Autodesk Inventor part; units mm, degrees
ref_plane "YZ Plane" through (0, 0, 0) normal (1, 0, 0) x (0, 1, 0)
ref_plane "XZ Plane" through (0, 0, 0) normal (0, 1, 0) x (-1, 0, 0)
ref_plane "XY Plane" through (0, 0, 0) normal (0, 0, 1) x (1, 0, 0)
sketch "Sketch1" plane through (0, 0, 0) normal (1, 0, 0) x (0, 1, 0)
  circle A0 centre (0, 0) radius 8.001
  dimension "d0" = 16.002
extrude "Extrusion1" add sketch "Sketch1" along normal blind 101.6254
sketch "Sketch2" plane through (101.6254, 0, 0) normal (1, 0, 0) x (0, 0, -1)
  line L0 (-6.2432, -5.0038) -> (6.2432, -5.0038)
  line L1 (-7.5991, -2.5038) -> (7.5991, -2.5038)
  arc A0 (6.2432, -5.0038) -> (7.5991, -2.5038) centre (0, 0) ccw
  arc A1 (-7.5991, -2.5038) -> (-6.2432, -5.0038) centre (0, 0) ccw
  circle A2 centre (0, 0) radius 8.001
  point P0 (7.0332, -3.8145)
  point P1 (-7.0332, -3.8145)
  dimension "d3" = 5.0038
  dimension "d4" = 2.5
extrude "Extrusion2" add sketch "Sketch2" along normal blind 22.86 contours A1 L1 A0 L0
sketch "Sketch3" plane through (101.6254, -2.5038, 7.5991) normal (0, 1, 0) x (1, 0, 0)
  circle A0 centre (15.2654, 7.5991) radius 4.1021
  line L0 (0, 15.1983) -> (22.86, 15.1983)
  line L1 (0, 0) -> (22.86, 0)
  line L2 (0, 0) -> (0, 15.1983)
  point P0 (-101.6254, 7.5991)
  dimension "d8" = 8.2042
  dimension "d9" = 7.5991
  dimension "d10" = 15.1983
  dimension "d13" = 15.2654
extrude "Extrusion3" cut sketch "Sketch3" against normal blind 15.0114
equation "\"d9\" = 0.5 * d10"
properties part number "Ring Connector model 5"
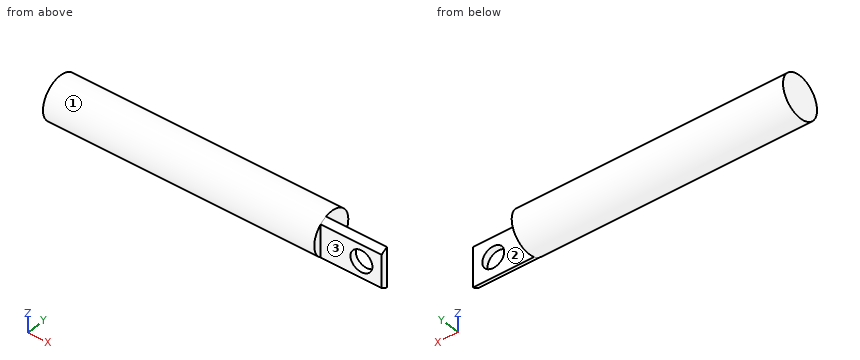
Geometry: final body of the model. Coordinates: model frame, mm. Face numbers are marked on the shaded views. A direction names the side the tool comes from. Give positions to 0.01 mm unless a question says otherwise; leave off trailing zeros. Write each loop counter-clockwise with the first axis right and the second up, starting at its lowest first coordinate (ties: lowest second). Pieces come first, ordered by that corner, then holes.
(1) First-contact query: P1, Ø7.5, axis at x = 117.5, z = 1.5, coming from the +Y side; P2, Ø1.5, axis at x = 65.5, z = 3.5, coming from the +Y side; P3, Ø2, axis at x = 12.5, y = -4, coming from the +Z side. Flat tips, straight axial feed; report the tip coordinate or a pass-through.
(2) Cut plane B-B, the plane x = 108. Return loops of the section in (y, z), then the cut area to 3 significant figures.
(3) Ray query, line 1 (X direction, y = -3.45, z = 0); line 2 (Z direction, x = 73, y = 5); line 3 (Z direction, x = 24.5, y = 0.5). Return the intervals inside material, ascending.
(4) Access query for the marked faces 1, 2 and 3. Directions: +Z, -Z, +X, -X, +Y, -Y. A direction counts if a zero-diameter tool reaches every point of the face in a straight line with its end or side. Return the directions, or none.
(5) Cut plane A-A, the plane z = 0. Return loops of the section in (x, y).
(6) Cut plane D-D, the plane x = 39. Return loops of the section in (y, z), then the cut area to 3 significant figures.
(7) Cut plane C-C, the plane y = 0. Return loops of the section in (x, z), then the cut area to 3 significant figures.
Values follow:
1. P1: stops at y = -2.5
1. P2: stops at y = 7.51
1. P3: stops at z = 7.42
2. outline: (-5, -6.24) arc R8 ccw to (-2.5, -7.6) - (-2.5, 7.6) arc R8 ccw to (-5, 6.24) - close
2. area: 35.1 mm2
3. line 1: x = 0 to 112.79, 120.99 to 124.49
3. line 2: z = -6.25 to 6.25
3. line 3: z = -7.99 to 7.99
4. face 1: +X, -X
4. face 2: +Z, -Z, +X, +Y
4. face 3: +Z, -Z, +X, -Y
5. outline: (0, -8) - (101.63, -8) - (101.63, -5) - (112.79, -5) - (112.79, -2.5) - (101.63, -2.5) - (101.63, 8) - (0, 8) - close; (120.99, -5) - (124.49, -5) - (124.49, -2.5) - (120.99, -2.5) - close
6. outline: circle Ø16 at (0, 0)
6. area: 201 mm2
7. outline: (0, -8) - (101.63, -8) - (101.63, 8) - (0, 8) - close
7. area: 1,630 mm2
